```python
from build123d import *

# Parameters (mm, degrees)
SKETCH1_R                              = 5.119071812
BOSS_EXTRUDE1_DEPTH                    = 10.16
F_97_0_0059_DIAMETER_HOLE1_D           = 0.14986
F_97_0_0059_DIAMETER_HOLE1_DEPTH       = 4.064
F_97_0_0059_DIAMETER_HOLE1_CSINK_D     = 3.0226
F_97_0_0059_DIAMETER_HOLE1_CSINK_ANGLE = 100
F_97_0_0059_DIAMETER_HOLE1_TIP         = 0.045022486
F_97_0_0059_DIAMETER_HOLE2_D           = 0.14986
F_97_0_0059_DIAMETER_HOLE2_DEPTH       = 4.064
F_97_0_0059_DIAMETER_HOLE2_CSINK_D     = 3.0226
F_97_0_0059_DIAMETER_HOLE2_CSINK_ANGLE = 100
F_97_0_0059_DIAMETER_HOLE2_TIP         = 0.045022486


with BuildPart() as part:
    # Sketch1 → Boss-Extrude1 (new body)
    with BuildSketch(Plane(origin=(0, 0, 0), x_dir=(0, 0, -1), z_dir=(1, 0, 0))):
        with Locations((-7.977955169, 45.822101484)):
            Circle(SKETCH1_R)
    extrude(amount=BOSS_EXTRUDE1_DEPTH)

    # #97 (0.0059) Diameter Hole1
    with Locations(Plane(origin=(10.16, 0, 0), x_dir=(0, 0, -1), z_dir=(1, 0, 0))):
        with Locations((-7.966953198, 45.502352874), (-8.184469296, 76.052039223), (-8.264751999, 76.50814273)):
            CounterSinkHole(F_97_0_0059_DIAMETER_HOLE1_D / 2, F_97_0_0059_DIAMETER_HOLE1_CSINK_D / 2, depth=F_97_0_0059_DIAMETER_HOLE1_DEPTH, counter_sink_angle=F_97_0_0059_DIAMETER_HOLE1_CSINK_ANGLE)
            with Locations((0, 0, -(F_97_0_0059_DIAMETER_HOLE1_DEPTH + F_97_0_0059_DIAMETER_HOLE1_TIP / 2))):  # 118° drill point
                Cone(0, F_97_0_0059_DIAMETER_HOLE1_D / 2, F_97_0_0059_DIAMETER_HOLE1_TIP, mode=Mode.SUBTRACT)

    # #97 (0.0059) Diameter Hole2
    with Locations(Plane.ZY):
        with Locations((8.054455303, 45.605487912), (7.835684071, 14.98353801)):
            CounterSinkHole(F_97_0_0059_DIAMETER_HOLE2_D / 2, F_97_0_0059_DIAMETER_HOLE2_CSINK_D / 2, depth=F_97_0_0059_DIAMETER_HOLE2_DEPTH, counter_sink_angle=F_97_0_0059_DIAMETER_HOLE2_CSINK_ANGLE)
            with Locations((0, 0, -(F_97_0_0059_DIAMETER_HOLE2_DEPTH + F_97_0_0059_DIAMETER_HOLE2_TIP / 2))):  # 118° drill point
                Cone(0, F_97_0_0059_DIAMETER_HOLE2_D / 2, F_97_0_0059_DIAMETER_HOLE2_TIP, mode=Mode.SUBTRACT)


solid = part.part
```
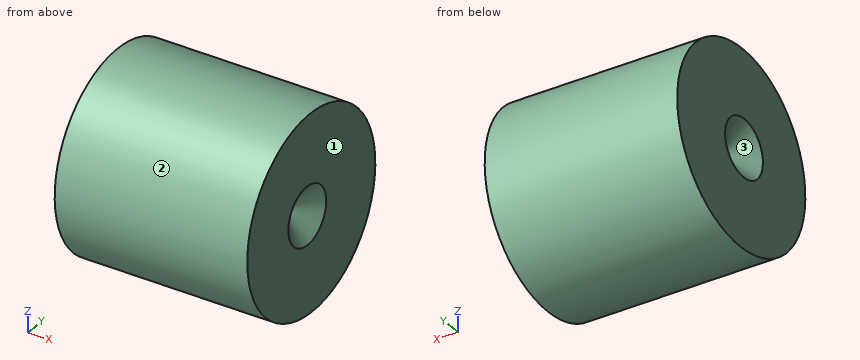
CAD build for the part. Positions are in the model's coordinates, mm. Face numbers are marked on the shaded views. Round coordinates to 2 decimals unless told otherwise and drop trailing zeros. Write each loop counter-clockwise with the first axis right and the second up, starting at its lowest first coordinate (ties: lowest second). Pieces come first, ordered by that corner, then holes. Notation, with made-up numbers: (22.25, 42.5) - (28.25, 42.5) arc R20 cw to (28.25, 53.5) - close; hole circle Ø4 at (-5.5, 42.5). An arc over 180 degrees is marked (long way). Return JSON: item names as keys, results as strings. Group by question number.
Item 1: Flat gauge pins, fed straight in: pin 1 Ø5 at (x, y) = (3.5, 42) entering from -Z; pin 2 Ø1.5 at (x, y) = (4, 47.5) entering from +Z; pin 3 Ø1.5 at (x, z) = (5, 6) entering from -Y. Where does each tip first touch, or does it go through?
Item 2: Band-saw the part on A-A on x = 9.25. List the corners of the cut face in (y, z), plus the area to 3 significant figures.
Item 3: Band-saw the part on D-D on x = 5.75. List the corners of the cut face in (y, z).
Item 4: Band-saw the part on C-C on z = 11. List the corners of the cut face in (x, y).
Item 5: Band-saw the part on B-B on y = 42.75. List the corners of the cut face in (x, z), plus the area to 3 significant figures.
Item 6: Probe probe 1 along Z at (x, y) = (9, 46); probe 2 along Y at (x, z) = (4.75, 7); probe 3 along Y at (x, z) = (9.25, 6.25). List the from-to ranges inside material, lowest first.
Item 7: Mould opens along Y. For the marked faces 1, 2 and 3 say: +Y half, -Y half, draft (parallel to the pull), parting line (faces both ways), or undercut.
Resolved:
{
 "1": {"pin 1": "stops at z = 3.03", "pin 2": "stops at z = 13.01", "pin 3": "stops at y = 40.85"},
 "2": {"outline": "circle Ø10.24 at (45.82, 7.98); hole circle Ø0.85 at (45.5, 7.97)", "area": "81.8 mm²"},
 "3": {"outline": "circle Ø10.24 at (45.82, 7.98)"},
 "4": {"outline": "(0, 41.69) - (10.16, 41.69) - (10.16, 49.95) - (0, 49.95) - close"},
 "5": {"outline": "(0, 3.88) - (10.16, 3.88) - (10.16, 12.07) - (0, 12.07) - close", "area": "83.2 mm²"},
 "6": {"probe 1": "z = 2.86 to 13.09", "probe 2": "y = 40.8 to 50.85", "probe 3": "y = 41 to 50.64"},
 "7": {"face 1": "draft", "face 2": "parting line", "face 3": "undercut"}
}
